Print and shaded views of the part. All mm, measured from the part's lowest x, y and z. Give positions to 0.01 mm unless a question says otherwise; leave off trailing zeros. Loops run counter-clockwise (first coordinate to the right, second up) from the corner with the lowest first, then second, coordinate; pieces in that order, holes last. Notation, with made-up numbers: M -39.75,61 L -8.75,61 A35 cw -8.75,97 Z; hole C 45.25,15.5 d2. An arc over 180 degrees is marked long. Answer as CSV lines item,"result".
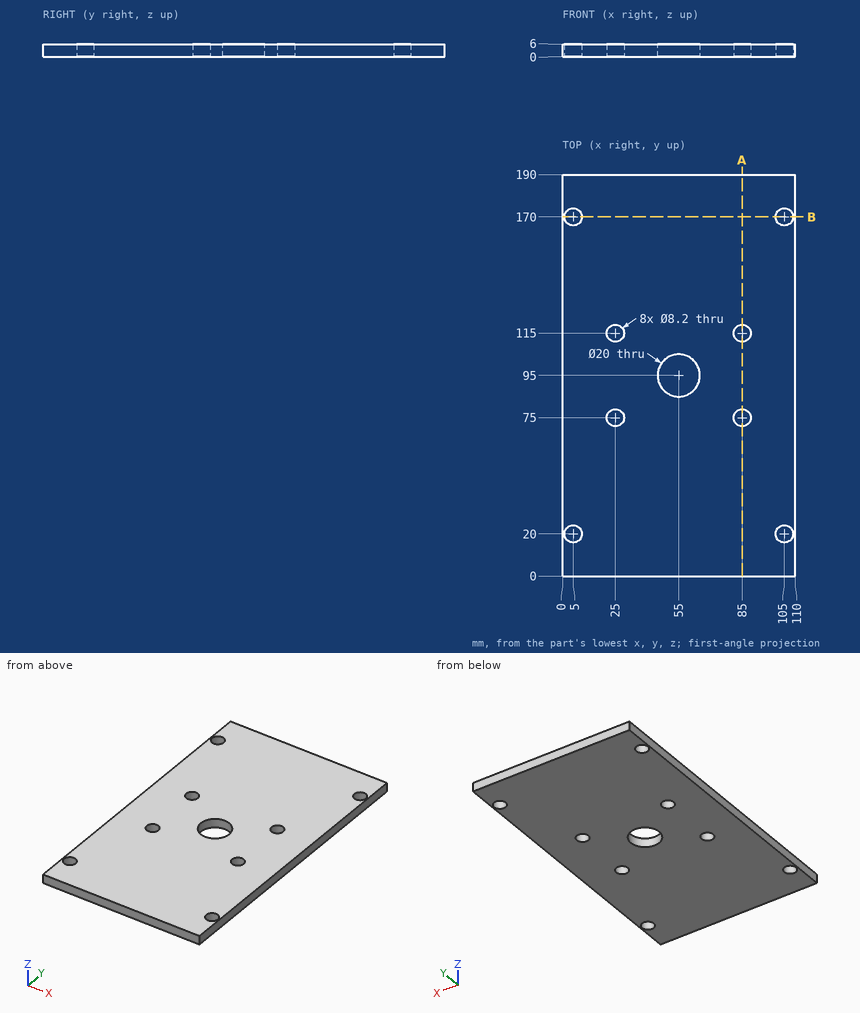
Q1. Wall check: line 1 (Y direction, x = 25, z = 2.75); line 2 (Y direction, x = 5, z = 3); line 3 (Y direction, x = 55, z = 3.5). Give the ranges that are in metal, low to high. Write a range as [from, to].
Solution:
line 1,"y = [0, 70.9], [79.1, 110.9], [119.1, 190]"
line 2,"y = [0, 15.9], [24.1, 165.9], [174.1, 190]"
line 3,"y = [0, 85], [105, 190]"
Q2. Cut at B-B (y = 170). Write the cut outline in (x, z), and give its area (3 significant figures).
Solution:
outline,"M 0,0 L 0.9,0 L 0.9,6 L 0,6 Z; M 9.1,0 L 100.9,0 L 100.9,6 L 9.1,6 Z; M 109.1,0 L 110,0 L 110,6 L 109.1,6 Z"
area,"562 mm²"
Q3. Pin check, flat tip, straight feed: P1, Ø3, axis at x = 33.5, z = 1.5, coming from the -Y side. Stop position of the tip, or through.
Solution:
P1,"stops at y = 0"
Q4. Cut at A-A (x = 85). Write the cut outline in (y, z), and give its area (3 significant figures).
Solution:
outline,"M 0,0 L 70.9,0 L 70.9,6 L 0,6 Z; M 79.1,0 L 110.9,0 L 110.9,6 L 79.1,6 Z; M 119.1,0 L 190,0 L 190,6 L 119.1,6 Z"
area,"1,040 mm²"
